```python
from build123d import *

# Parameters (mm, degrees)
ESQUISSE1_R = 5


with BuildPart() as part:
    # Balayage1: sweep along a path in Esquisse2
    with BuildLine(Plane(origin=(0, 0, 0), x_dir=(0, 0, -1), z_dir=(1, 0, 0))) as balayage1_path:
        Line((-150, -300), (-150, -10))
        ThreePointArc((-150, -10), (-147.071067812, -2.928932188), (-140, 0))
        Line((-140, 0), (140, 0))
        ThreePointArc((140, 0), (147.071067812, -2.928932188), (150, -10))
        Line((150, -10), (150, -300))
    # Esquisse1 → Balayage1 (sweep)
    with BuildSketch(Plane.XY):
        Circle(ESQUISSE1_R)
    sweep(path=balayage1_path.line)


solid = part.part
```
Can you work these out from the model? Positions are in its coordinate system, mm. A direction names the side the tool comes from. Round coordinates to 2 decimals unless told otherwise and drop trailing zeros. Loops run counter-clockwise (first coordinate to the right, second up) from the corner with the lowest first, then second, coordinate; pieces in that order, holes last. Notation, with made-up numbers: M 43.5,-5.75 L 90.5,-5.75 A26 ccw 90.5,32.25 Z; hole C -39,0 d1. An arc over 180 degrees is marked long. Write item = value, one per line. Start each with the question number.
(1) Suppose I cut it at C-C on z = 111.5. Write out the boundary of the cut face in (x, y).
(2) Suppose I cut it at B-B on y = -55. Write out the boundary of the cut face in (x, z), plus the area to 3 significant figures.
(3) If we mould it in two halves opening along Z, with no side actions, what happens to faces 3 (the face through (-1.08, -152.97, 154.88)), 4 (the face through (0, -300, -150)), 5 (the face through (-1.08, 4.88, -1.96))? For each: released by +Z, released by -Z, zero draft, split by the parting line, or undercut.
(4) Which directions (+Z, -Z, +X, -X, +Y, -Y) give clear straight access to the entire face, cutting with the end or side of a thin tool? Please do faces 1 (the face through (-1.08, -157.03, -154.88)), 2 (the face through (0, -300, 150)).
(5) I need wall thicknesses on line 1 along Z through (x, y) = (0, -85.5); line 2 along Z through (x, y) = (1.75, -99); line 3 along Y through (x, z) = (0, 61). Which ranges of each line are inside material? Lowest first, please.
(6) Suppose I cut it at A-A on x = 0. Write out the boundary of the cut face in (y, z).
(7) I'm going to push flat-ended pins straight in: P1, Ø2, axis at x = -4, y = -139, coming from the +Z side; P2, Ø1.5, axis at x = 4, z = -47, coming from the -Y side; P3, Ø1, axis at x = 2, y = -195, coming from the -Z side. Where does each tip first touch, or does it pass through?
Answer block:
q1.outline = C 0,0 d10
q2.outline = C 0,-150 d10; C 0,150 d10
q2.area = 157 mm²
q3.face_3 = undercut
q3.face_4 = zero draft
q3.face_5 = undercut
q4.face_1 = -Y
q4.face_2 = +Z, -Z, +X, -X, -Y
q5.line_1 = -155 to -145, 145 to 155
q5.line_2 = -154.68 to -145.32, 145.32 to 154.68
q5.line_3 = -5 to 5
q6.outline = M -300,-155 L -10,-155 A15 ccw 5,-140 L 5,140 A15 ccw -10,155 L -300,155 L -300,145 L -10,145 A5 cw -5,140 L -5,-140 A5 cw -10,-145 L -300,-145 Z
q7.P1 = 154
q7.P2 = -3.8
q7.P3 = -154.77
